```python
from build123d import *

# Parameters (mm, degrees)
SKIZZE1_W                       = 25
SKIZZE1_H                       = 8
AUFSATZ_LINEAR_AUSTRAGEN1_DEPTH = 124
SKIZZE2_W                       = 2
SKIZZE2_H                       = 6.8
SCHNITT_LINEAR_AUSTRAGEN1_DEPTH = 135.693866119
SKIZZE3_R                       = 1.75
SKIZZE3_W                       = 6
SKIZZE3_H                       = 6
SCHNITT_LINEAR_AUSTRAGEN2_DEPTH = 131.739829541
SKIZZE4_W                       = 4
SKIZZE4_H                       = 6.8
SCHNITT_LINEAR_AUSTRAGEN3_DEPTH = 1.2
SKIZZE5_R                       = 2
SKIZZE5_R_2                     = 4
SCHNITT_LINEAR_AUSTRAGEN4_DEPTH = 131.739829541
LINEARES_MUSTER1_COUNT          = 11
LINEARES_MUSTER1_PITCH          = 10
SKIZZE6_W                       = 90.5
SKIZZE6_H                       = 21
SCHNITT_LINEAR_AUSTRAGEN5_DEPTH = 6
SKIZZE7_W                       = 33.5
SKIZZE7_H                       = 13
SCHNITT_LINEAR_AUSTRAGEN6_DEPTH = 6
SKIZZE8_W                       = 7.2
SKIZZE8_H                       = 6
AUFSATZ_LINEAR_AUSTRAGEN2_DEPTH = 6
AUFSATZ_LINEAR_AUSTRAGEN3_REACH = 132.633
SKIZZE9_W                       = 1.5
SKIZZE9_H                       = 3
FASE1_SIZE                      = 1.5


with BuildPart() as part:
    # Skizze1 → Aufsatz-Linear austragen1 (new body)
    with BuildSketch(Plane(origin=(0, 0, 0), x_dir=(0, 0, -1), z_dir=(1, 0, 0))):
        with Locations((-28.15591013, -29.369664989)):
            Rectangle(SKIZZE1_W, SKIZZE1_H)
    extrude(amount=AUFSATZ_LINEAR_AUSTRAGEN1_DEPTH)

    # Skizze2 → Schnitt-Linear austragen1 (cut, through all)
    with BuildSketch(Plane.ZY):
        with Locations((16.65591013, -28.769664989)):
            Rectangle(SKIZZE2_W, SKIZZE2_H)
        with Locations((39.65591013, -28.769664989)):
            Rectangle(SKIZZE2_W, SKIZZE2_H)
    extrude(amount=-SCHNITT_LINEAR_AUSTRAGEN1_DEPTH, mode=Mode.SUBTRACT)

    # Skizze3 → Schnitt-Linear austragen2 (cut, through all)
    with BuildSketch(Plane(origin=(0, -25.369664989, 0), x_dir=(1, 0, 0), z_dir=(0, 1, 0))):
        with Locations(Location((121.15, -28.15591013, 0), (0, 0, 270))):
            Circle(SKIZZE3_R)
        with Locations((121, -18.65591013)):
            Rectangle(SKIZZE3_W, SKIZZE3_H)
        with Locations((121, -37.65591013)):
            Rectangle(SKIZZE3_W, SKIZZE3_H)
    extrude(amount=-SCHNITT_LINEAR_AUSTRAGEN2_DEPTH, mode=Mode.SUBTRACT)

    # Skizze4 → Schnitt-Linear austragen3 (cut)
    with BuildSketch(Plane(origin=(118, 0, 0), x_dir=(0, 0, -1), z_dir=(1, 0, 0))):
        with Locations((-36.65591013, -28.769664989)):
            Rectangle(SKIZZE4_W, SKIZZE4_H)
        with Locations((-19.65591013, -28.769664989)):
            Rectangle(SKIZZE4_W, SKIZZE4_H)
    extrude(amount=-SCHNITT_LINEAR_AUSTRAGEN3_DEPTH, mode=Mode.SUBTRACT)

    # Skizze5 → Schnitt-Linear austragen4 (cut, through all)
    with BuildSketch(Plane(origin=(0, -25.369664989, 0), x_dir=(1, 0, 0), z_dir=(0, 1, 0))):
        with Locations(Location((3, -20.65591013, 0), (0, 0, 270))):
            Circle(SKIZZE5_R)
        with Locations(Location((5, -28.15591013, 0), (0, 0, 270))):
            Circle(SKIZZE5_R_2)
        with Locations(Location((3, -35.65591013, 0), (0, 0, 270))):
            Circle(SKIZZE5_R)
        with Locations(Location((8, -35.65591013, 0), (0, 0, 270))):
            Circle(SKIZZE5_R)
        with Locations(Location((8, -20.65591013, 0), (0, 0, 270))):
            Circle(SKIZZE5_R)
    schnitt_linear_austragen4 = extrude(amount=-SCHNITT_LINEAR_AUSTRAGEN4_DEPTH, mode=Mode.SUBTRACT)

    # Lineares Muster1: Schnitt-Linear austragen4 ×11
    with Locations(*[(i * LINEARES_MUSTER1_PITCH, 0, 0) for i in range(1, LINEARES_MUSTER1_COUNT)]):
        add(schnitt_linear_austragen4, mode=Mode.SUBTRACT)

    # Skizze6 → Schnitt-Linear austragen5 (cut)
    with BuildSketch(Plane(origin=(0, -25.369664989, 0), x_dir=(1, 0, 0), z_dir=(0, 1, 0))):
        with Locations((45.25, -28.15591013)):
            Rectangle(SKIZZE6_W, SKIZZE6_H)
    extrude(amount=-SCHNITT_LINEAR_AUSTRAGEN5_DEPTH, mode=Mode.SUBTRACT)

    # Skizze7 → Schnitt-Linear austragen6 (cut)
    with BuildSketch(Plane.XZ.offset(33.369664989)):
        with Locations((107.25, 28.15591013)):
            Rectangle(SKIZZE7_W, SKIZZE7_H)
    extrude(amount=-SCHNITT_LINEAR_AUSTRAGEN6_DEPTH, mode=Mode.SUBTRACT)

    # Skizze8 → Aufsatz-Linear austragen2 (add)
    with BuildSketch(Plane(origin=(0, -25.369664989, 0), x_dir=(1, 0, 0), z_dir=(0, 1, 0))):
        with Locations((120.4, -18.65591013)):
            Rectangle(SKIZZE8_W, SKIZZE8_H)
        with Locations((120.4, -37.65591013)):
            Rectangle(SKIZZE8_W, SKIZZE8_H)
    extrude(amount=-AUFSATZ_LINEAR_AUSTRAGEN2_DEPTH)

    # Aufsatz-Linear austragen3: up to this face of the body (flat: up to its plane)
    aufsatz_linear_austragen3_end = Plane(part.part.faces().sort_by_distance((110.417879916, -25.369664989, 28.15591013))[0])
    # Skizze9 → Aufsatz-Linear austragen3 (add, up to the picked face)
    with BuildSketch(Plane(origin=(0, -31.369664989, 0), x_dir=(1, 0, 0), z_dir=(0, 1, 0)), mode=Mode.PRIVATE) as aufsatz_linear_austragen3_sk1:
        with Locations((89.75, -28.15591013)):
            Rectangle(SKIZZE9_W, SKIZZE9_H)
    aufsatz_linear_austragen3_tool1 = split(extrude(aufsatz_linear_austragen3_sk1.sketch, amount=AUFSATZ_LINEAR_AUSTRAGEN3_REACH, mode=Mode.PRIVATE), bisect_by=aufsatz_linear_austragen3_end, keep=Keep.BOTH, mode=Mode.PRIVATE)
    add(aufsatz_linear_austragen3_tool1.solids().sort_by(Axis((89.75, -31.369665, 28.15591), (0, 1, 0)))[0])

    # Fase1
    fase1_edges = [part.edges().sort_by_distance(p)[0] for p in [
        (90.5, -26.369664989, 29.65591013),
        (90.5, -26.369664989, 26.65591013),
    ]]
    chamfer(fase1_edges, length=FASE1_SIZE - 0.0001)  # a hair under: the kernel refuses the full size


solid = part.part
```
Can you work these out from the model? Positions are in its coordinate system, mm. Coordinates: 2 decimals unless noted, no trailing zeros. Loops run counter-clockwise (first coordinate to the right, second up) from the corner with the lowest first, then second, coordinate; pieces in that order, holes last.
1) Imagine slicing it at A-A on x = 23. List the corners of the cut face in (y, z) for me.
2) I need wall thicknesses on probe 1 along Z at (x, y) = (108, -29); probe 2 along X at (y, z) = (-29.75, 37.25); probe 3 along X at (y, z) = (-29.75, 19). Which ranges of each line are inside material? Lowest first, please.
3) For pin 1 (1.8 mm diameter, centred on x = 81, z = 17.5, fed in from +Y); pin 2 (4.5 mm diameter, centred on x = 93, z = 20.66, fed in from -Y); pin 3 (1.5 mm diameter, centred on x = 101.5, y = -31, fed in from +Z); pin 4 (1.6 mm diameter, centred on y = -27.5, z = 17, fed in from -X), each with a flat end and sliding along its axis, tell me the tip position at first contact or that it passes through.
4) Thinking about a two-plate mould opening in X: for faces 1 (the flat face through (110, -27.37, 28)), 2 (the flat face through (89, -28, 28)), 3 (the cylindrical face through (64.686, -32.356, 36.731)), 4 (the cylindrical face through (14.35, -32.36, 34.18)), which applies, pulls with the +X half, pulls with the -X half, needs draft (parallel to the pull), parting line crosses it, or undercut?
5) Imagine slicing it at B-B on z = 19.75. State how many separate pieces and enclosed holes the cut face has, plus the area to 3 significant figures.
Completed:
1. outline: (-33.37, 15.66) - (-32.17, 15.66) - (-32.17, 17.66) - (-31.37, 17.66) - (-31.37, 18.66) - (-33.37, 18.66) - close; (-33.37, 22.66) - (-31.37, 22.66) - (-31.37, 24.69) - (-33.37, 24.69) - close; (-33.37, 31.62) - (-31.37, 31.62) - (-31.37, 33.66) - (-33.37, 33.66) - close; (-33.37, 37.66) - (-31.37, 37.66) - (-31.37, 38.66) - (-32.17, 38.66) - (-32.17, 40.66) - (-33.37, 40.66) - close
2. probe 1: z = 17.66 to 18.66, 37.66 to 38.66
2. probe 2: x = 90.5 to 91.79, 94.21 to 96.79, 99.21 to 101.79, 104.21 to 106.79, 109.21 to 124
2. probe 3: x = 90.5 to 91.88, 94.12 to 96.88, 99.12 to 101.88, 104.12 to 106.88, 109.12 to 124
3. pin 1: stops at y = -31.37
3. pin 2: stops at y = -33.37
3. pin 3: stops at z = 38.66
3. pin 4: stops at x = 90.5
4. face 1: needs draft
4. face 2: pulls with the -X half
4. face 3: undercut
4. face 4: undercut
5. separate pieces: 23
5. enclosed holes: 0
5. area: 194 mm2
